Read the model definition and answer for the solid it produces. Units are mm, in the model's axes. Face numbers are marked on the shaded views. A direction names the side the tool comes from. Coordinates: 2 decimals unless noted, no trailing zeros. Write each loop counter-clockwise with the first axis right and the second up, starting at its lowest first coordinate (ties: lowest second). Pieces come first, ordered by that corner, then holes. Notation, with made-up numbers: M 0.25,-6.5 L 5.25,-6.5 A15 cw 5.25,0.5 Z; hole C -28.75,-38.75 d4. An arc over 180 degrees is marked long. Use a Markdown table: item, result. Add a question column.
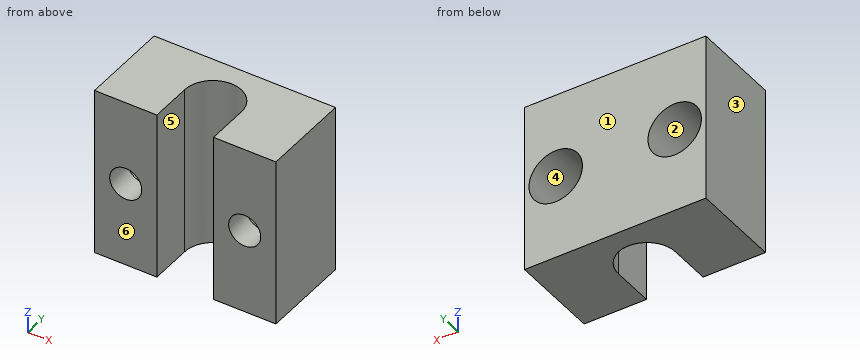
from build123d import *

# Parameters (mm, degrees)
BOSS_EXTRUDE1_DEPTH = 19
SKETCH2_R           = 1.8
CUT_EXTRUDE1_DEPTH  = 24.836170519
SKETCH2_3_R         = 3
SKETCH2_3_R_2       = 1.8
CUT_EXTRUDE2_DEPTH  = 7.18


with BuildPart() as part:
    # Sketch1 → Boss-Extrude1 (new body)
    with BuildSketch(Plane.XY):
        with BuildLine():
            Line((-10.175, 0), (-10.175, 10.18))
            Line((-10.175, 10.18), (10.175, 10.18))
            Line((10.175, 10.18), (10.175, 0))
            Line((10.175, 0), (3.175, 0))
            Line((3.175, 0), (3.175, 4.75))
            ThreePointArc((3.175, 4.75), (0, 7.925), (-3.175, 4.75))
            Line((-3.175, 4.75), (-3.175, 0))
            Line((-3.175, 0), (-10.175, 0))
        make_face()
    extrude(amount=BOSS_EXTRUDE1_DEPTH)

    # Sketch2 → Cut-Extrude1 (cut, through all)
    with BuildSketch(Plane(origin=(0, 10.18, 0), x_dir=(1, 0, 0), z_dir=(0, 1, 0))):
        with Locations(Location((-6.675, -9.5, 0), (0, 0, 270))):
            Circle(SKETCH2_R)
        with Locations(Location((6.675, -9.5, 0), (0, 0, 270))):
            Circle(SKETCH2_R)
    extrude(amount=-CUT_EXTRUDE1_DEPTH, mode=Mode.SUBTRACT)

    # Sketch2<3> → Cut-Extrude2 (cut)
    # profile 1 of 2: a face of its own
    with BuildSketch(Plane(origin=(0, 10.18, 0), x_dir=(1, 0, 0), z_dir=(0, 1, 0))):
        with Locations(Location((-6.675, -9.5, 0), (0, 0, 270))):
            Circle(SKETCH2_3_R)
        with Locations(Location((-6.675, -9.5, 0), (0, 0, 270))):
            Circle(SKETCH2_3_R_2, mode=Mode.SUBTRACT)
    # profile 2 of 2: a face of its own
    with BuildSketch(Plane(origin=(0, 10.18, 0), x_dir=(1, 0, 0), z_dir=(0, 1, 0))):
        with Locations(Location((6.675, -9.5, 0), (0, 0, 270))):
            Circle(SKETCH2_3_R)
    extrude(amount=-CUT_EXTRUDE2_DEPTH, mode=Mode.SUBTRACT)


solid = part.part
Item 1: Find section D-D on z = 16. Give the vertices of the cut face in (x, y) (3 decimals), then the cut area to 3 significant figures.
Item 2: Each of these flat-tipped pins is pushed along its axis until it touches: pin 1 (1.8 mm diameter, centred on x = 6, z = 10.5, fed in from +Y); pin 2 (1 mm diameter, centred on x = 0.5, z = 2.5, fed in from -Y). Where does it stop, or does it pass through?
Item 3: Find section B-B on z = 9.5. Give the vertices of the cut face in (x, y) (3 decimals), then the cut area to 3 significant figures.
Item 4: Find section C-C on x = 7.5. Give the vertices of the cut face in (y, z).
Item 5: For the marked faces 4, 5 and 6, determine the directions among +Z, -Z, +X, -X, +Y, -Y from which every point of the face is accessible in a straight line to the end or side of a thin tool.
Item 6: Determine the mould class of the marked faces 1, 2 and 3 for opening direction X: pulls with the +X half, pulls with the -X half, needs draft (parallel to the pull), parting line crosses it, or undercut.
Item 7: Find section A-A on y = 7. Give the vertices of the cut face in (x, z) (3 decimals), then the cut area to 3 significant figures.
Item 8: Consider probe 1 along X at (y, z) = (1.65, 9.5) (3 decimals); probe 2 along X at (y, z) = (5.75, 8) (3 decimals); probe 3 along X at (y, z) = (4, 3.75) (3 decimals). Determine where each line is inside the solid, lowest interval first.
Geometry says:
| question | item | result |
|---|---|---|
| 1 | outline | M -10.175,0 L -3.175,0 L -3.175,4.75 A3.175 cw 3.175,4.75 L 3.175,0 L 10.175,0 L 10.175,10.18 L -10.175,10.18 Z |
| 1 | area | 161 mm2 |
| 2 | pin 1 | stops at y = 3 |
| 2 | pin 2 | stops at y = 7.76 |
| 3 | outline | M -10.175,0 L -8.475,0 L -8.475,3 L -9.675,3 L -9.675,10.18 L -10.175,10.18 Z; M -4.875,0 L -3.175,0 L -3.175,4.75 A3.175 cw 3.175,4.75 L 3.175,0 L 4.875,0 L 4.875,3 L 3.675,3 L 3.675,10.18 L -3.675,10.18 L -3.675,3 L -4.875,3 Z; M 8.475,0 L 10.175,0 L 10.175,10.18 L 9.675,10.18 L 9.675,3 L 8.475,3 Z |
| 3 | area | 53.4 mm2 |
| 4 | outline | M 0,0 L 10.18,0 L 10.18,6.62 L 3,6.62 L 3,7.9 L 0,7.9 Z; M 0,11.1 L 3,11.1 L 3,12.38 L 10.18,12.38 L 10.18,19 L 0,19 Z |
| 5 | face 4 | +Y |
| 5 | face 5 | +Z, -Z, -Y |
| 5 | face 6 | +Z, -Z, +X, -X, -Y |
| 6 | face 1 | needs draft |
| 6 | face 2 | undercut |
| 6 | face 3 | pulls with the -X half |
| 7 | outline | M -10.175,0 L -2.24,0 L -2.24,19 L -10.175,19 Z; M 2.24,0 L 10.175,0 L 10.175,19 L 2.24,19 Z; hole C -6.675,9.5 d6; hole C 6.675,9.5 d6 |
| 7 | area | 245 mm2 |
| 8 | probe 1 | x = -10.175 to -8.475, -4.875 to -3.175, 3.175 to 4.875, 8.475 to 10.175 |
| 8 | probe 2 | x = -10.175 to -9.273, -4.077 to -3.013, 3.013 to 4.077, 9.273 to 10.175 |
| 8 | probe 3 | x = -10.175 to -3.175, 3.175 to 10.175 |
